```python
from build123d import *

# Parameters (mm, degrees)
F0_W     = 137.48005
F0_H     = 26.821588
F1_DEPTH = 12.192
F2_SIZE  = 2.54
F3_R     = 2.54


with BuildPart() as f1:
    # F0 (on Top) → F1 (new body)
    with BuildSketch(Plane.XY):
        with BuildLine():
            Line((-68.740025, -13.410794), (-68.740025, 13.410794))
            ThreePointArc((-68.740025, 13.410794), (-82.150819, 0), (-68.740025, -13.410794))
        make_face()
        Rectangle(F0_W, F0_H)
        Polygon((87.603755, 13.410794), (68.740025, 13.410794), (68.740025, -13.410794), align=None)
    extrude(amount=F1_DEPTH)

    # F2
    f2_edges = [f1.edges().sort_by_distance(p)[0] for p in [
        (9.431865, 13.410794, 12.192),
        (-82.150819, 0, 12.192),
        (0, -13.410794, 12.192),
        (78.17189, 0, 12.192),
    ]]
    chamfer(f2_edges, length=F2_SIZE)

    # F3
    f3_edges = [f1.edges().sort_by_distance(p)[0] for p in [
        (87.603755, 13.410794, 4.826),
    ]]
    fillet(f3_edges, radius=F3_R)


solid = f1.part
```
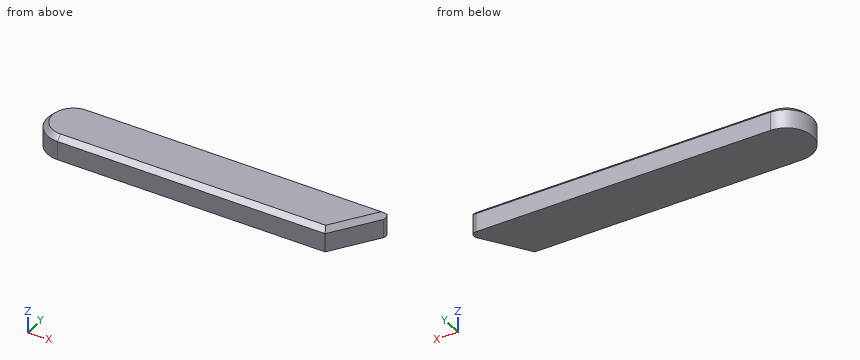
Read the model definition and answer for the solid it produces. Units are mm, in the model's axes. Coordinates: 2 decimals unless noted, no trailing zeros. Loops run counter-clockwise (first coordinate to the right, second up) from the corner with the lowest first, then second, coordinate; pieces in that order, holes last. Notation, with made-up numbers: (1, -34) -> (13, -34) arc R32 ccw to (13, 1) -> close; hole circle Ø8 at (-17, 48). An arc over 180 degrees is marked (long way). Return JSON: item names as keys, results as strings.
Item 1: A flat-ended cylindrical pin translates along its axis: P1, Ø1.5, axis at y = -2.5, z = 9.5, coming from the -X side. Find the tip coordinate at first contact, or state that the pin passes through.
Answers:
{"P1": "stops at x = -82.04"}
Item 2: Find section A-A (z = 3.5). Determine the outline of the cut face in (x, y), plus the area to 3 significant figures.
Answers:
{"outline": "(-68.74, -13.41) -> (68.74, -13.41) -> (84.79, 9.41) arc R2.54 ccw to (82.71, 13.41) -> (-68.74, 13.41) arc R13.41 ccw to start", "area": "4,220 mm2"}
Item 3: Find the intervals of material crossed by probe 1 along Y at (x, z) = (-69.5, 1.25); probe 2 along X at (y, z) = (-1, 9); probe 3 along X at (y, z) = (-11.25, 10.5), in increasing order.
Answers:
{"probe 1": "y = -13.39 to 13.39", "probe 2": "x = -82.11 to 77.47", "probe 3": "x = -74.33 to 69.22"}
Item 4: Find section B-B (x = 61). Determine the outline of the cut face in (y, z).
Answers:
{"outline": "(-13.41, 0) -> (13.41, 0) -> (13.41, 9.65) -> (10.87, 12.19) -> (-10.87, 12.19) -> (-13.41, 9.65) -> close"}
Item 5: Find section C-C (y = 0). Determine the outline of the cut face in (x, z), plus the area to 3 significant figures.
Answers:
{"outline": "(-82.15, 0) -> (78.17, 0) -> (78.17, 9.65) -> (75.07, 12.19) -> (-79.61, 12.19) -> (-82.15, 9.65) -> close", "area": "1,950 mm2"}
